Geometry check sheet. Reference: the model listing, model coordinates, mm. Round coordinates to 2 decimals unless told otherwise and drop trailing zeros. Write each loop counter-clockwise with the first axis right and the second up, starting at its lowest first coordinate (ties: lowest second). Pieces come first, ordered by that corner, then holes. Notation, with made-up numbers: M 3.25,76 L 44.25,76 A29 ccw 44.25,109 Z; hole C 75,45.25 d6. An arc over 180 degrees is marked long. One line per item, written item: value. Start each with the question number.
1. Section check A-A (z = -76.5). Record the boundary of the cut face in (x, y) (3 decimals).
2. Section check C-C (x = 0.7). Record the boundary of the cut face in (y, z) (3 decimals).
3. Section check D-D (y = 69.85). Record the boundary of the cut face in (x, z) (3 decimals), and give its area (3 significant figures).
4. Section check B-B (y = -7). Record the boundary of the cut face in (x, z) (3 decimals), and give its area (3 significant figures).
5. Scan lines: probe 1 along Y at (x, z) = (1.55, -60.5); probe 2 along Y at (x, z) = (1.8, -80); probe 3 along Z at (x, y) = (1.95, -6.5). Record each from-to range of solid material in increasing order. Write a range as [from, to].
from build123d import *

# Parameters (mm, degrees)
SKETCH1_W           = 152.4
SKETCH1_H           = 165.1
BOSS_EXTRUDE1_DEPTH = 3.175
CUT_EXTRUDE1_DEPTH  = 4.175
SKETCH3_R           = 3.175
CUT_EXTRUDE2_DEPTH  = 4.175


with BuildPart() as part:
    # Sketch1 → Boss-Extrude1 (new body)
    with BuildSketch(Plane(origin=(0, 0, 0), x_dir=(0, 0, -1), z_dir=(1, 0, 0))):
        with Locations((76.2, 0)):
            Rectangle(SKETCH1_W, SKETCH1_H)
    extrude(amount=BOSS_EXTRUDE1_DEPTH)

    # Sketch2 → Cut-Extrude1 (cut, through all)
    with BuildSketch(Plane.ZY):
        with BuildLine():
            Line((-107.95, 25.4), (-107.95, -25.4))
            ThreePointArc((-107.95, -25.4), (-106.090128061, -29.890128061), (-101.6, -31.75))
            Line((-101.6, -31.75), (-50.8, -31.75))
            ThreePointArc((-50.8, -31.75), (-46.309871939, -29.890128061), (-44.45, -25.4))
            Line((-44.45, -25.4), (-44.45, 25.4))
            ThreePointArc((-44.45, 25.4), (-46.309871939, 29.890128061), (-50.8, 31.75))
            Line((-50.8, 31.75), (-101.6, 31.75))
            ThreePointArc((-101.6, 31.75), (-106.090128061, 29.890128061), (-107.95, 25.4))
        make_face()
    extrude(amount=-CUT_EXTRUDE1_DEPTH, mode=Mode.SUBTRACT)

    # Sketch3 → Cut-Extrude2 (cut, through all)
    with BuildSketch(Plane.ZY):
        with Locations((-60.325, 69.85)):
            Circle(SKETCH3_R)
        with Locations((-92.075, 69.85)):
            Circle(SKETCH3_R)
        with Locations((-92.075, -69.85)):
            Circle(SKETCH3_R)
        with Locations((-60.325, -69.85)):
            Circle(SKETCH3_R)
    extrude(amount=-CUT_EXTRUDE2_DEPTH, mode=Mode.SUBTRACT)


solid = part.part
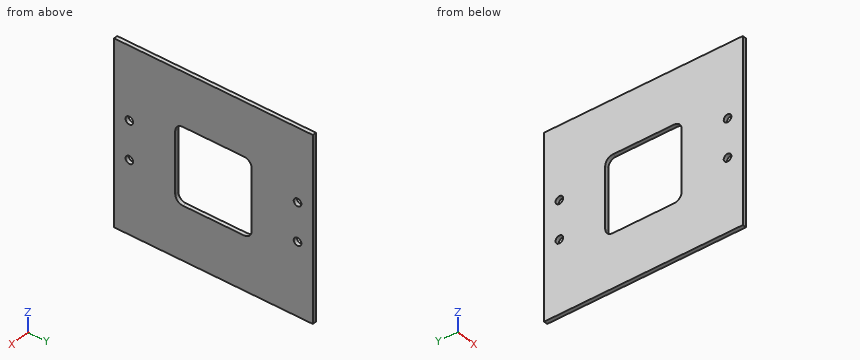
Result sheet:
1. outline: M 0,-82.55 L 3.175,-82.55 L 3.175,-31.75 L 0,-31.75 Z; M 0,31.75 L 3.175,31.75 L 3.175,82.55 L 0,82.55 Z
2. outline: M -82.55,-152.4 L 82.55,-152.4 L 82.55,0 L -82.55,0 Z; hole C -69.85,-92.075 d6.35; hole C -69.85,-60.325 d6.35; hole M -31.75,-101.6 A6.35 ccw -25.4,-107.95 L 25.4,-107.95 A6.35 ccw 31.75,-101.6 L 31.75,-50.8 A6.35 ccw 25.4,-44.45 L -25.4,-44.45 A6.35 ccw -31.75,-50.8 Z; hole C 69.85,-92.075 d6.35; hole C 69.85,-60.325 d6.35
3. outline: M 0,-152.4 L 3.175,-152.4 L 3.175,-95.25 L 0,-95.25 Z; M 0,-88.9 L 3.175,-88.9 L 3.175,-63.5 L 0,-63.5 Z; M 0,-57.15 L 3.175,-57.15 L 3.175,0 L 0,0 Z
3. area: 444 mm2
4. outline: M 0,-152.4 L 3.175,-152.4 L 3.175,-107.95 L 0,-107.95 Z; M 0,-44.45 L 3.175,-44.45 L 3.175,0 L 0,0 Z
4. area: 282 mm2
5. probe 1: y = [-82.55, -73.02], [-66.68, -31.75], [31.75, 66.68], [73.02, 82.55]
5. probe 2: y = [-82.55, -31.75], [31.75, 82.55]
5. probe 3: z = [-152.4, -107.95], [-44.45, 0]
